Design review of the part built by this model. Coordinates are the model's own, in mm. Coordinates: 2 decimals unless noted, no trailing zeros. Write each loop counter-clockwise with the first axis right and the second up, starting at its lowest first coordinate (ties: lowest second). Pieces come first, ordered by that corner, then holes. Notation, with made-up numbers: (-5.5, 20.5) - (50.5, 20.5) arc R20 cw to (50.5, 40.5) - close; hole circle Ø8 at (13, -37). An arc over 180 degrees is marked (long way). Answer as a JSON object with one key per item and string values.
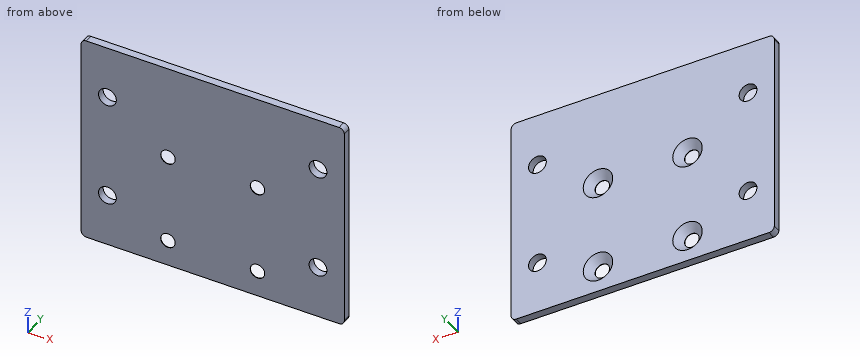
```python
from build123d import *

# Parameters (mm, degrees)
CROQUIS1_W                                   = 100
CROQUIS1_H                                   = 80
BRIDA_BASE1_DEPTH                            = 3
REDONDEO1_R                                  = 2
TALADRO_DE_MARGEN_PARA_1_41_D                = 6.7564
REFRENTADO_PARA_TORNILLO_TAP_N_CON_C_2_COUNT = 2
REFRENTADO_PARA_TORNILLO_TAP_N_CON_C_2_PITCH = 34
REFRENTADO_PARA_TORNILLO_TAP_N_CON_C_3_COUNT = 2
REFRENTADO_PARA_TORNILLO_TAP_N_CON_C_3_PITCH = 48.083261121
REFRENTADO_PARA_TORNILLO_TAP_N_CON_C_4_COUNT = 2
REFRENTADO_PARA_TORNILLO_TAP_N_CON_C_4_PITCH = 34


# Sheet-metal steps are written as plain solids
with BuildPart() as part:
    # Croquis1 → Brida base1 (new body)
    with BuildSketch(Plane(origin=(0, 0, 0), x_dir=(1, 0, 0), z_dir=(0, 1, 0))):
        with Locations((-99.777777778, -5.555555556)):
            Rectangle(CROQUIS1_W, CROQUIS1_H)
    extrude(amount=-BRIDA_BASE1_DEPTH)

    # Redondeo1
    redondeo1_edges = [part.edges().sort_by_distance(p)[0] for p in [
        (-149.777777778, -1.5, -34.444444444),
        (-49.777777778, -1.5, -34.444444444),
        (-49.777777778, -1.5, 45.555555556),
        (-149.777777778, -1.5, 45.555555556),
    ]]
    fillet(redondeo1_edges, radius=REDONDEO1_R)

    # Taladro de margen para 1/41 (through all)
    with Locations(Plane(origin=(0, 0, 0), x_dir=(1, 0, 0), z_dir=(0, 1, 0))):
        with Locations((-139.777777778, -25.555555556), (-59.777777778, -25.555555556), (-139.777777778, 14.444444444), (-59.777777778, 14.444444444)):
            Hole(TALADRO_DE_MARGEN_PARA_1_41_D / 2)

    # Croquis9 → Refrentado para tornillo tapón con cabeza plana de clavija de M51 (revolve, cut)
    with BuildSketch(Plane(origin=(-116.777777778, 0, -24.444444444), x_dir=(0, 0, 1), z_dir=(1, 0, 0))):
        Polygon((0, 0), (0, 3), (2.75, 3), (2.75, 2.85), (5.6, 0), align=None)
    refrentado_para_tornillo_tap_n_con_cabez = revolve(axis=Axis((-116.777777778, 6.35, -24.444444444), (0, -1, 0)), mode=Mode.SUBTRACT)

    # Refrentado para tornillo tap_n con c 2: Refrentado para tornillo tapón con cabeza plana de clavija de M51 ×2
    with Locations(*[(i * REFRENTADO_PARA_TORNILLO_TAP_N_CON_C_2_PITCH, 0, 0) for i in range(1, REFRENTADO_PARA_TORNILLO_TAP_N_CON_C_2_COUNT)]):
        add(refrentado_para_tornillo_tap_n_con_cabez, mode=Mode.SUBTRACT)

    # Refrentado para tornillo tap_n con c 3: Refrentado para tornillo tapón con cabeza plana de clavija de M51 ×2
    with Locations(*[Vector(0.7071067811865476, 0, 0.7071067811865476) * (i * REFRENTADO_PARA_TORNILLO_TAP_N_CON_C_3_PITCH) for i in range(1, REFRENTADO_PARA_TORNILLO_TAP_N_CON_C_3_COUNT)]):
        add(refrentado_para_tornillo_tap_n_con_cabez, mode=Mode.SUBTRACT)

    # Refrentado para tornillo tap_n con c 4: Refrentado para tornillo tapón con cabeza plana de clavija de M51 ×2
    with Locations(*[(0, 0, i * REFRENTADO_PARA_TORNILLO_TAP_N_CON_C_4_PITCH) for i in range(1, REFRENTADO_PARA_TORNILLO_TAP_N_CON_C_4_COUNT)]):
        add(refrentado_para_tornillo_tap_n_con_cabez, mode=Mode.SUBTRACT)


solid = part.part
```
(1) To check wall thickness, follow line 1 (X direction, y = -0.45, z = 23.5); line 2 (Z direction, x = -139, y = -2.2); line 3 (Z direction, x = -141, y = -1.6). State the ranges of each line that lie inside material, in increasing order. Write a range as from..to.
Solved:
{"line 1": "x = -149.78..-142.46, -137.1..-62.46, -57.1..-49.78", "line 2": "z = -34.44..-17.73, -11.16..22.27, 28.84..45.56", "line 3": "z = -34.44..-17.59, -11.3..22.41, 28.7..45.56"}
(2) Take a section at A-A, the plane y = -2.2. Give the number of separate pieces and of enclosed holes in the cut face, and give its area (3 significant figures).
Solved:
{"separate pieces": "1", "enclosed holes": "8", "area": "7,710 mm^2"}
(3) For pin 1 (6 mm diameter, centred on x = -114, z = 33, fed in from +Y); pin 2 (7 mm diameter, centred on x = -116.78, z = -24.44, fed in from +Y); pin 3 (9 mm diameter, centred on x = -82.78, z = -24.44, fed in from +Y), all flat-tipped, find the tip position at first contact; note any pin that passes through.
Solved:
{"pin 1": "stops at y = 0", "pin 2": "stops at y = -2.1", "pin 3": "stops at y = -1.1"}
(4) Take a section at B-B, the plane z = 24. Write out the cut boundary in (x, y).
Solved:
{"outline": "(-149.78, -3) - (-142.78, -3) - (-142.78, 0) - (-149.78, 0) - close; (-136.78, -3) - (-62.78, -3) - (-62.78, 0) - (-136.78, 0) - close; (-56.78, -3) - (-49.78, -3) - (-49.78, 0) - (-56.78, 0) - close"}
(5) Take a section at C-C, the plane x = -62. Write out the cut boundary in (y, z).
Solved:
{"outline": "(-3, -34.44) - (0, -34.44) - (0, -16.99) - (-3, -16.99) - close; (-3, -11.9) - (0, -11.9) - (0, 23.01) - (-3, 23.01) - close; (-3, 28.1) - (0, 28.1) - (0, 45.56) - (-3, 45.56) - close"}
